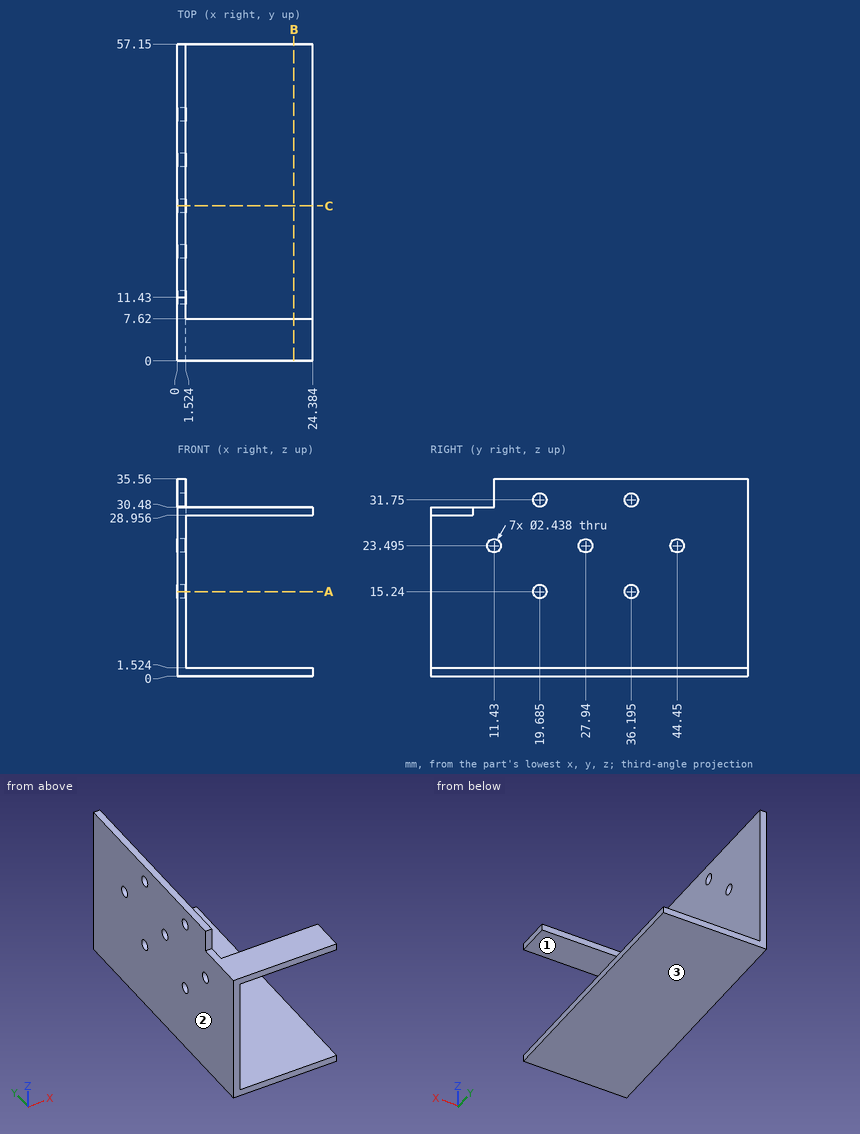
Print and shaded views of the part. All mm, measured from the part's lowest x, y and z. Round coordinates to 2 decimals unless told otherwise and drop trailing zeros. Write each loop counter-clockwise with the first axis right and the second up, starting at its lowest first coordinate (ties: lowest second). Pieces come first, ordered by that corner, then holes.
(1) Probe line 1 along Z through (x, y) = (8, 7.5); line 2 along X through (y, z) = (54, 3). List the from-to ranges inside material, lowest first.
(2) Slice it at C-C, the plane y = 27.94. Write the cut outline in (x, z) (1 decimal).
(3) Slice it at B-B, the plane x = 21. Write the cut outline in (y, z).
(4) Mould opens along Z. For the marked faces 1, 2 and 3 say: pulls with the +Z half, pulls with the -Z half, needs draft (parallel to the pull), parting line crosses it, or undercut.
(5) Drop flat-ended pins along their axis: P1, Ø1.2, axis at x = 0.5, z = 32, coming from the -Y side; P2, Ø3, axis at y = 19.685, z = 31.75, coming from the +X side; P3, Ø1.7, axis at x = 10.5, z = 29.5, coming from the +Y side. Give the stop position or say it passes through.
(6) Slice it at A-A, the plane z = 15.24. Count the separate pieces of the cut face and the enclosed holes in it.
From the geometry:
1. line 1: z = 0 to 1.52, 28.96 to 30.48
1. line 2: x = 0 to 1.52
2. outline: (0, 0) - (24.4, 0) - (24.4, 1.5) - (1.5, 1.5) - (1.5, 22.3) - (0, 22.3) - close; (0, 24.7) - (1.5, 24.7) - (1.5, 35.6) - (0, 35.6) - close
3. outline: (0, 0) - (57.15, 0) - (57.15, 1.52) - (0, 1.52) - close; (0, 28.96) - (7.62, 28.96) - (7.62, 30.48) - (0, 30.48) - close
4. face 1: undercut
4. face 2: needs draft
4. face 3: pulls with the -Z half
5. P1: stops at y = 11.43
5. P2: stops at x = 1.52
5. P3: stops at y = 7.62
6. separate pieces: 3
6. enclosed holes: 0
